from build123d import *

# Parameters (mm, degrees)
SALIENTE_EXTRUIR1_DEPTH = 10
CROQUIS2_R              = 5
SALIENTE_EXTRUIR2_DEPTH = 100
SALIENTE_EXTRUIR3_DEPTH = 10
CROQUIS4_W              = 10
CROQUIS4_H              = 10
SALIENTE_EXTRUIR4_DEPTH = 50
CROQUIS5_R              = 5
CORTAR_EXTRUIR1_DEPTH   = 0.1


with BuildPart() as part:
    # Croquis1 → Saliente-Extruir1 (new body)
    with BuildSketch(Plane.XY):
        with BuildLine():
            Line((-150, 10), (150, 10))
            ThreePointArc((150, 10), (160, 0), (150, -10))
            Line((150, -10), (-150, -10))
            ThreePointArc((-150, -10), (-160, 0), (-150, 10))
        make_face()
    extrude(amount=SALIENTE_EXTRUIR1_DEPTH)

    # Croquis2 → Saliente-Extruir2 (add)
    with BuildSketch(Plane.XY.offset(10)):
        with Locations((-150, 0)):
            Circle(CROQUIS2_R)
    extrude(amount=SALIENTE_EXTRUIR2_DEPTH)

    # Croquis3 → Saliente-Extruir3 (add)
    with BuildSketch(Plane.XY.offset(110)):
        with BuildLine():
            Line((-150, -10), (150, -10))
            ThreePointArc((150, -10), (160, 0), (150, 10))
            Line((150, 10), (-150, 10))
            ThreePointArc((-150, 10), (-160, 0), (-150, -10))
        make_face()
    extrude(amount=SALIENTE_EXTRUIR3_DEPTH)

    # Croquis4 → Saliente-Extruir4 (add)
    with BuildSketch(Plane.XZ.offset(10)):
        with Locations((-145, 115)):
            Rectangle(CROQUIS4_W, CROQUIS4_H)
        with Locations((145, 115)):
            Rectangle(CROQUIS4_W, CROQUIS4_H)
        with Locations((145, 5)):
            Rectangle(CROQUIS4_W, CROQUIS4_H)
        with Locations((-145, 5)):
            Rectangle(CROQUIS4_W, CROQUIS4_H)
    extrude(amount=SALIENTE_EXTRUIR4_DEPTH)

    # Croquis5 → Cortar-Extruir1 (cut)
    with BuildSketch(Plane.XY.offset(10)):
        with Locations((150, 0)):
            Circle(CROQUIS5_R)
    extrude(amount=-CORTAR_EXTRUIR1_DEPTH, mode=Mode.SUBTRACT)


solid = part.part
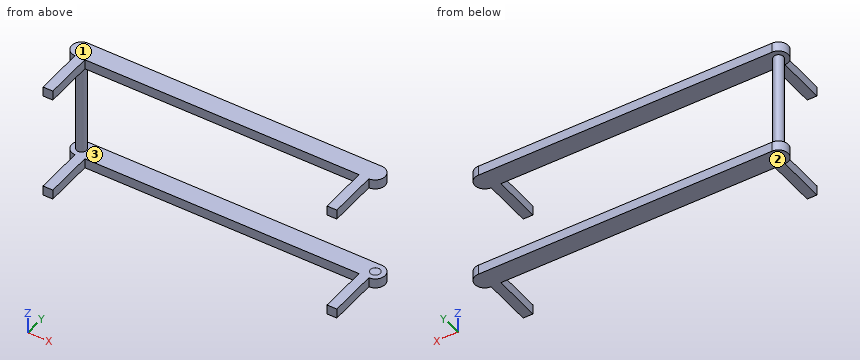
The model under review builds one solid part; all positions refer to its coordinate system, in mm. Face numbers are marked on the shaded views. Round coordinates to 2 decimals unless told otherwise and drop trailing zeros. Loops run counter-clockwise (first coordinate to the right, second up) from the corner with the lowest first, then second, coordinate; pieces in that order, holes last. Notation, with made-up numbers: (13.25, 22) - (31.25, 22) arc R26 cw to (31.25, 60) - close; hole circle Ø4 at (73.25, -21.75). An arc over 180 degrees is marked (long way). Use CSV: the item, a comma, the result in double quotes.
(1) Take a section at A-A, the plane y = -39. Give the boundary of the cut face in (x, z).
Working result:
outline,"(-150, 0) - (-140, 0) - (-140, 10) - (-150, 10) - close; (-150, 110) - (-140, 110) - (-140, 120) - (-150, 120) - close; (140, 0) - (150, 0) - (150, 10) - (140, 10) - close; (140, 110) - (150, 110) - (150, 120) - (140, 120) - close"
(2) Take a section at D-D, the plane z = 102.5. Give the boundary of the cut face in (x, y), plus the area to 3 significant figures.
Working result:
outline,"circle Ø10 at (-150, 0)"
area,"78.5 mm^2"
(3) For line 1 (Z direction, x = 10.5, y = 1.5); line 2 (Y direction, x = 34.5, z = 5.5); line 3 (X direction, y = 0, z = 9), list the stretches that pass through material, from the lowest coordinate up.
Working result:
line 1,"z = 0 to 10, 110 to 120"
line 2,"y = -10 to 10"
line 3,"x = -160 to 160"
(4) Take a section at B-B, the plane x = 133.5. Give the boundary of the cut face in (y, z).
Working result:
outline,"(-10, 0) - (10, 0) - (10, 10) - (-10, 10) - close; (-10, 110) - (10, 110) - (10, 120) - (-10, 120) - close"
(5) Take a section at C-C, the plane y = 0. Give the boundary of the cut face in (x, z).
Working result:
outline,"(-160, 0) - (160, 0) - (160, 10) - (155, 10) - (155, 9.9) - (145, 9.9) - (145, 10) - (-145, 10) - (-145, 110) - (160, 110) - (160, 120) - (-160, 120) - (-160, 110) - (-155, 110) - (-155, 10) - (-160, 10) - close"
(6) Clearance check with flat-ended pins moving along their axes: P1, Ø11, axis at y = -42.5, z = 7, coming from the +X side; P2, Ø11, axis at y = -31.5, z = 114.5, coming from the -X side; P3, Ø5, axis at x = -14.5, z = 112.5, coming from the -Y side. State where each tip first meets the part, or that it passes through.
Working result:
P1,"stops at x = 150"
P2,"stops at x = -150"
P3,"stops at y = -10"
(7) The part is to be moulded in two halves that separate along Z. For the marked faces 1, 2 and 3, say which applies: pulls with the +Z half, pulls with the -Z half, needs draft (parallel to the pull), parting line crosses it, or undercut.
Working result:
face 1,"pulls with the +Z half"
face 2,"pulls with the -Z half"
face 3,"undercut"
